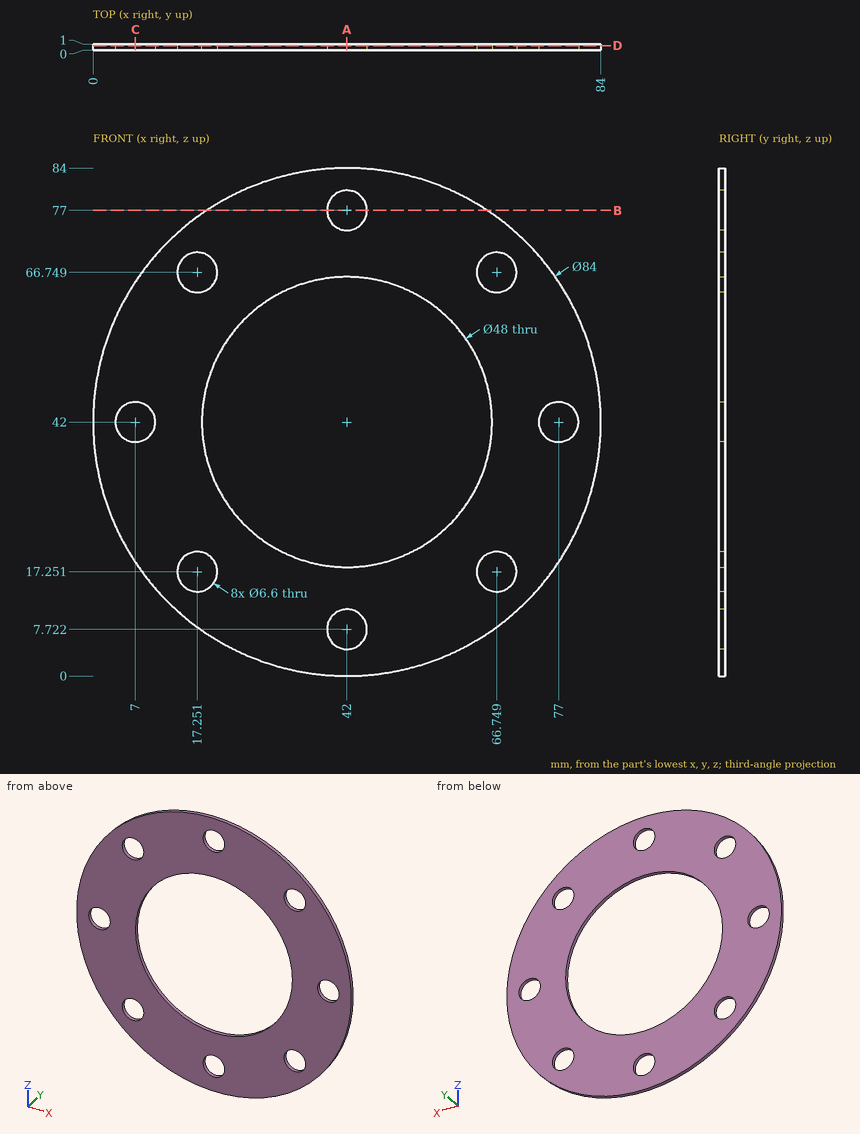
Could you check a few things on this drawing? It's one solid part, dimensions in mm from its lowest x, y, z. Coordinates: 2 decimals unless noted, no trailing zeros. Write each loop counter-clockwise with the first axis right and the second up, starting at its lowest first coordinate (ties: lowest second). Pieces come first, ordered by that corner, then holes.
Q1. Imagine slicing it at D-D, the plane y = 0.75. Count the separate pieces of the cut face and the enclosed holes in it, plus the area to 3 significant figures.
Results found:
separate pieces: 1
enclosed holes: 9
area: 3,460 mm2
Q2. Imagine slicing it at C-C, the plane x = 7. List the corners of the cut face in (y, z) for me.
Results found:
outline: (0, 18.78) - (1, 18.78) - (1, 38.7) - (0, 38.7) - close; (0, 45.3) - (1, 45.3) - (1, 65.22) - (0, 65.22) - close
Q3. Imagine slicing it at A-A, the plane x = 42. List the corners of the cut face in (y, z) for me, plus the area to 3 significant figures.
Results found:
outline: (0, 0) - (1, 0) - (1, 4.42) - (0, 4.42) - close; (0, 11.02) - (1, 11.02) - (1, 18) - (0, 18) - close; (0, 66) - (1, 66) - (1, 73.7) - (0, 73.7) - close; (0, 80.3) - (1, 80.3) - (1, 84) - (0, 84) - close
area: 22.8 mm2
Q4. Please list where these lines run through material, in increasing order: L1, parallel to Z at x = 42, y = 0.4; L2, parallel to Z at x = 17.5, y = 0.1 (1 decimal); L3, parallel to Z at x = 75, y = 0.45 (1 decimal).
Results found:
L1: z = 0 to 4.42, 11.02 to 18, 66 to 73.7, 80.3 to 84
L2: z = 7.9 to 14, 20.5 to 63.5, 70 to 76.1
L3: z = 16 to 39.4, 44.6 to 68
Q5. Imagine slicing it at B-B, the plane z = 77. List the corners of the cut face in (x, y) for me.
Results found:
outline: (18.78, 0) - (38.7, 0) - (38.7, 1) - (18.78, 1) - close; (45.3, 0) - (65.22, 0) - (65.22, 1) - (45.3, 1) - close
